```python
from build123d import *

# Parameters (mm, degrees)
F0_W     = 47.244
F0_H     = 31.496
F1_DEPTH = 3.20802
F2_R     = 2.4638
F3_DEPTH = 1.7526


with BuildPart() as f1:
    # F0 (on Top) → F1 (new body)
    with BuildSketch(Plane.XY):
        Rectangle(F0_W, F0_H)
    extrude(amount=F1_DEPTH)

    # F2 (on face) → F3 (join)
    with BuildSketch(Plane.XY.offset(3.20802)):
        with BuildLine():
            ThreePointArc((-17.2212, 11.811), (-21.4271696875, 13.5531696875), (-19.685, 9.3472))
            ThreePointArc((-19.685, 9.3472), (-17.9428303125, 10.0688303125), (-17.2212, 11.811))
        make_face()
        with Locations((-11.811, 11.811)):
            Circle(F2_R)
        with BuildLine():
            Line((-3.937, 11.811), (-3.937, 9.3472))
            ThreePointArc((-3.937, 9.3472), (-2.1948303125, 10.0688303125), (-1.4732, 11.811))
            ThreePointArc((-1.4732, 11.811), (-3.937, 14.2748), (-6.4008, 11.811))
            Line((-6.4008, 11.811), (-3.937, 11.811))
        make_face()
        with BuildLine():
            ThreePointArc((-6.4008, 11.811), (-5.6791696875, 10.0688303125), (-3.937, 9.3472))
            Line((-3.937, 9.3472), (-3.937, 11.811))
            Line((-3.937, 11.811), (-6.4008, 11.811))
        make_face()
        with BuildLine():
            ThreePointArc((6.4008, 11.811), (2.1948303125, 13.5531696875), (3.937, 9.3472))
            Line((3.937, 9.3472), (3.937, 11.811))
            Line((3.937, 11.811), (6.4008, 11.811))
        make_face()
        with BuildLine():
            Line((3.937, 11.811), (3.937, 9.3472))
            ThreePointArc((3.937, 9.3472), (5.6791696875, 10.0688303125), (6.4008, 11.811))
            Line((6.4008, 11.811), (3.937, 11.811))
        make_face()
        with BuildLine():
            Line((3.937, 3.937), (3.937, 1.4732))
            ThreePointArc((3.937, 1.4732), (5.6791696875, 2.1948303125), (6.4008, 3.937))
            ThreePointArc((6.4008, 3.937), (5.6791696875, 5.6791696875), (3.937, 6.4008))
            Line((3.937, 6.4008), (3.937, 3.937))
        make_face()
        with BuildLine():
            ThreePointArc((3.937, 6.4008), (1.4732, 3.937), (3.937, 1.4732))
            Line((3.937, 1.4732), (3.937, 3.937))
            Line((3.937, 3.937), (3.937, 6.4008))
        make_face()
        with BuildLine():
            Line((-3.937, 3.937), (-6.4008, 3.937))
            ThreePointArc((-6.4008, 3.937), (-3.937, 1.4732), (-1.4732, 3.937))
            ThreePointArc((-1.4732, 3.937), (-2.1948303125, 5.6791696875), (-3.937, 6.4008))
            Line((-3.937, 6.4008), (-3.937, 3.937))
        make_face()
        with BuildLine():
            ThreePointArc((-3.937, 6.4008), (-5.6791696875, 5.6791696875), (-6.4008, 3.937))
            Line((-6.4008, 3.937), (-3.937, 3.937))
            Line((-3.937, 3.937), (-3.937, 6.4008))
        make_face()
        with BuildLine():
            ThreePointArc((-9.3472, 3.937), (-11.811, 6.4008), (-14.2748, 3.937))
            Line((-14.2748, 3.937), (-11.811, 3.937))
            Line((-11.811, 3.937), (-9.3472, 3.937))
        make_face()
        with BuildLine():
            Line((-11.811, 3.937), (-14.2748, 3.937))
            ThreePointArc((-14.2748, 3.937), (-11.811, 1.4732), (-9.3472, 3.937))
            Line((-9.3472, 3.937), (-11.811, 3.937))
        make_face()
        with BuildLine():
            Line((-19.685, 6.4008), (-19.685, 3.937))
            Line((-19.685, 3.937), (-17.2212, 3.937))
            ThreePointArc((-17.2212, 3.937), (-17.9428303125, 5.6791696875), (-19.685, 6.4008))
        make_face()
        with BuildLine():
            Line((-19.685, 3.937), (-19.685, 1.4732))
            ThreePointArc((-19.685, 1.4732), (-17.9428303125, 2.1948303125), (-17.2212, 3.937))
            Line((-17.2212, 3.937), (-19.685, 3.937))
        make_face()
        with BuildLine():
            ThreePointArc((-19.685, 6.4008), (-22.1488, 3.937), (-19.685, 1.4732))
            Line((-19.685, 1.4732), (-19.685, 3.937))
            Line((-19.685, 3.937), (-19.685, 6.4008))
        make_face()
        with BuildLine():
            ThreePointArc((-17.2212, -3.937), (-17.9428303125, -2.1948303125), (-19.685, -1.4732))
            Line((-19.685, -1.4732), (-19.685, -3.937))
            Line((-19.685, -3.937), (-17.2212, -3.937))
        make_face()
        with BuildLine():
            Line((-17.2212, -3.937), (-19.685, -3.937))
            Line((-19.685, -3.937), (-19.685, -6.4008))
            ThreePointArc((-19.685, -6.4008), (-17.9428303125, -5.6791696875), (-17.2212, -3.937))
        make_face()
        with BuildLine():
            Line((-19.685, -3.937), (-19.685, -1.4732))
            ThreePointArc((-19.685, -1.4732), (-22.1488, -3.937), (-19.685, -6.4008))
            Line((-19.685, -6.4008), (-19.685, -3.937))
        make_face()
        with BuildLine():
            ThreePointArc((-9.3472, -3.937), (-11.811, -1.4732), (-14.2748, -3.937))
            Line((-14.2748, -3.937), (-11.811, -3.937))
            Line((-11.811, -3.937), (-9.3472, -3.937))
        make_face()
        with BuildLine():
            Line((-11.811, -3.937), (-14.2748, -3.937))
            ThreePointArc((-14.2748, -3.937), (-11.811, -6.4008), (-9.3472, -3.937))
            Line((-9.3472, -3.937), (-11.811, -3.937))
        make_face()
        with BuildLine():
            Line((-3.937, -3.937), (-6.4008, -3.937))
            ThreePointArc((-6.4008, -3.937), (-5.6791696875, -5.6791696875), (-3.937, -6.4008))
            Line((-3.937, -6.4008), (-3.937, -3.937))
        make_face()
        with BuildLine():
            ThreePointArc((-1.4732, -3.937), (-3.937, -1.4732), (-6.4008, -3.937))
            Line((-6.4008, -3.937), (-3.937, -3.937))
            Line((-3.937, -3.937), (-3.937, -6.4008))
            ThreePointArc((-3.937, -6.4008), (-2.1948303125, -5.6791696875), (-1.4732, -3.937))
        make_face()
        with BuildLine():
            ThreePointArc((-1.4732, -11.811), (-2.1948303125, -10.0688303125), (-3.937, -9.3472))
            Line((-3.937, -9.3472), (-3.937, -11.811))
            Line((-3.937, -11.811), (-6.4008, -11.811))
            ThreePointArc((-6.4008, -11.811), (-3.937, -14.2748), (-1.4732, -11.811))
        make_face()
        with BuildLine():
            Line((-3.937, -11.811), (-3.937, -9.3472))
            ThreePointArc((-3.937, -9.3472), (-5.6791696875, -10.0688303125), (-6.4008, -11.811))
            Line((-6.4008, -11.811), (-3.937, -11.811))
        make_face()
        with Locations((-11.811, -11.811)):
            Circle(F2_R)
        with BuildLine():
            ThreePointArc((-17.2212, -11.811), (-17.9428303125, -10.0688303125), (-19.685, -9.3472))
            ThreePointArc((-19.685, -9.3472), (-21.4271696875, -13.5531696875), (-17.2212, -11.811))
        make_face()
        with BuildLine():
            Line((3.937, -11.811), (3.937, -9.3472))
            ThreePointArc((3.937, -9.3472), (2.1948303125, -13.5531696875), (6.4008, -11.811))
            Line((6.4008, -11.811), (3.937, -11.811))
        make_face()
        with BuildLine():
            ThreePointArc((6.4008, -11.811), (5.6791696875, -10.0688303125), (3.937, -9.3472))
            Line((3.937, -9.3472), (3.937, -11.811))
            Line((3.937, -11.811), (6.4008, -11.811))
        make_face()
        with BuildLine():
            ThreePointArc((6.4008, -3.937), (5.6791696875, -2.1948303125), (3.937, -1.4732))
            Line((3.937, -1.4732), (3.937, -3.937))
            Line((3.937, -3.937), (3.937, -6.4008))
            ThreePointArc((3.937, -6.4008), (5.6791696875, -5.6791696875), (6.4008, -3.937))
        make_face()
        with BuildLine():
            Line((3.937, -3.937), (3.937, -1.4732))
            ThreePointArc((3.937, -1.4732), (1.4732, -3.937), (3.937, -6.4008))
            Line((3.937, -6.4008), (3.937, -3.937))
        make_face()
        with Locations((11.811, -3.937)):
            Circle(F2_R)
        with BuildLine():
            Line((19.685, -3.937), (19.685, -6.4008))
            ThreePointArc((19.685, -6.4008), (21.4271696875, -5.6791696875), (22.1488, -3.937))
            ThreePointArc((22.1488, -3.937), (19.685, -1.4732), (17.2212, -3.937))
            Line((17.2212, -3.937), (19.685, -3.937))
        make_face()
        with BuildLine():
            ThreePointArc((17.2212, -3.937), (17.9428303125, -5.6791696875), (19.685, -6.4008))
            Line((19.685, -6.4008), (19.685, -3.937))
            Line((19.685, -3.937), (17.2212, -3.937))
        make_face()
        with BuildLine():
            Line((19.685, -11.811), (17.2212, -11.811))
            ThreePointArc((17.2212, -11.811), (19.685, -14.2748), (22.1488, -11.811))
            ThreePointArc((22.1488, -11.811), (21.4271696875, -10.0688303125), (19.685, -9.3472))
            Line((19.685, -9.3472), (19.685, -11.811))
        make_face()
        with BuildLine():
            ThreePointArc((19.685, -9.3472), (17.9428303125, -10.0688303125), (17.2212, -11.811))
            Line((17.2212, -11.811), (19.685, -11.811))
            Line((19.685, -11.811), (19.685, -9.3472))
        make_face()
        with BuildLine():
            ThreePointArc((14.2748, -11.811), (11.811, -9.3472), (9.3472, -11.811))
            Line((9.3472, -11.811), (11.811, -11.811))
            Line((11.811, -11.811), (14.2748, -11.811))
        make_face()
        with BuildLine():
            Line((11.811, -11.811), (9.3472, -11.811))
            ThreePointArc((9.3472, -11.811), (11.811, -14.2748), (14.2748, -11.811))
            Line((14.2748, -11.811), (11.811, -11.811))
        make_face()
        with BuildLine():
            ThreePointArc((22.1488, 3.937), (21.4271696875, 5.6791696875), (19.685, 6.4008))
            Line((19.685, 6.4008), (19.685, 3.937))
            Line((19.685, 3.937), (17.2212, 3.937))
            ThreePointArc((17.2212, 3.937), (19.685, 1.4732), (22.1488, 3.937))
        make_face()
        with BuildLine():
            Line((19.685, 3.937), (19.685, 6.4008))
            ThreePointArc((19.685, 6.4008), (17.9428303125, 5.6791696875), (17.2212, 3.937))
            Line((17.2212, 3.937), (19.685, 3.937))
        make_face()
        with Locations((11.811, 3.937)):
            Circle(F2_R)
        with BuildLine():
            Line((11.811, 11.811), (9.3472, 11.811))
            ThreePointArc((9.3472, 11.811), (11.811, 9.3472), (14.2748, 11.811))
            Line((14.2748, 11.811), (11.811, 11.811))
        make_face()
        with BuildLine():
            ThreePointArc((14.2748, 11.811), (11.811, 14.2748), (9.3472, 11.811))
            Line((9.3472, 11.811), (11.811, 11.811))
            Line((11.811, 11.811), (14.2748, 11.811))
        make_face()
        with BuildLine():
            ThreePointArc((22.1488, 11.811), (19.685, 14.2748), (17.2212, 11.811))
            Line((17.2212, 11.811), (19.685, 11.811))
            Line((19.685, 11.811), (19.685, 9.3472))
            ThreePointArc((19.685, 9.3472), (21.4271696875, 10.0688303125), (22.1488, 11.811))
        make_face()
        with BuildLine():
            Line((19.685, 11.811), (17.2212, 11.811))
            ThreePointArc((17.2212, 11.811), (17.9428303125, 10.0688303125), (19.685, 9.3472))
            Line((19.685, 9.3472), (19.685, 11.811))
        make_face()
    extrude(amount=F3_DEPTH)


solid = f1.part
```
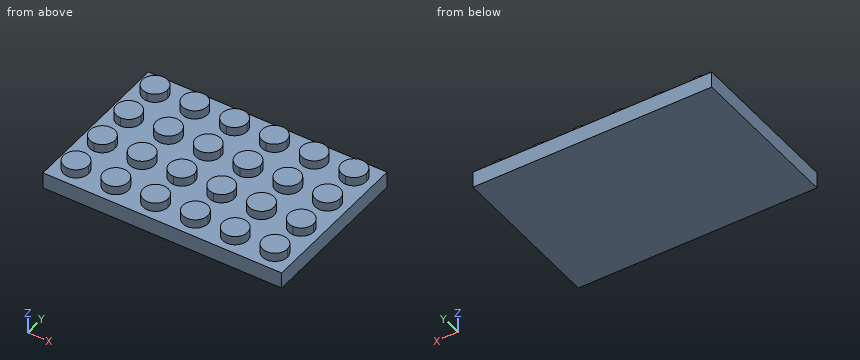
Here's how the part is built. I have some questions about the finished solid (model axes, mm). Give positions to 0.01 mm unless a question says otherwise; leave off trailing zeros. Order: outer loops, then holes, each group sorted by start corner. A loop starts at its lowest first (then second) coordinate and runs counter-clockwise, first axis right, second up. Notation, with made-up numbers: M -24.5,15.25 L -4.5,15.25 A22 ccw -4.5,50.25 Z; hole C 5,19.5 d7. An arc over 180 degrees is marked long. Use a Markdown table: item, result. Add a question column.
1. I need wall thicknesses on probe 1 along X at (y, z) = (12, 4.25); probe 2 along X at (y, z) = (-10, 4.5); probe 3 along Y at (x, z) = (-19, 3.3). Which ranges of each line are inside material? Lowest first, please. Write a range as from..to.
2. Suppose I cut it at D-D (x = -10). List the corners of the cut face in (y, z) for me, and give its area (3 significant figures).
3. Suppose I cut it at B-B (z = 3.9). Give the number of separate pieces and of enclosed holes in the cut face, and give its area (3 significant figures).
4. Suppose I cut it at C-C (y = -5). List the corners of the cut face in (x, z) for me, and give its area (3 significant figures).
5. Suppose I cut it at A-A (x = -3). List the corners of the cut face in (y, z) for me, and give its area (3 significant figures).
Results list:
| question | item | result |
|---|---|---|
| 1 | probe 1 | x = -22.14..-17.23, -14.27..-9.35, -6.39..-1.48, 1.48..6.39, 9.35..14.27, 17.23..22.14 |
| 1 | probe 2 | x = -21.36..-18.01, -13.48..-10.14, -5.61..-2.27, 2.27..5.61, 10.14..13.48, 18.01..21.36 |
| 1 | probe 3 | y = -14.18..-9.44, -6.3..-1.57, 1.57..6.3, 9.44..14.18 |
| 2 | outline | M -15.75,0 L 15.75,0 L 15.75,3.21 L 13.48,3.21 L 13.48,4.96 L 10.14,4.96 L 10.14,3.21 L 5.61,3.21 L 5.61,4.96 L 2.27,4.96 L 2.27,3.21 L -2.27,3.21 L -2.27,4.96 L -5.61,4.96 L -5.61,3.21 L -10.14,3.21 L -10.14,4.96 L -13.48,4.96 L -13.48,3.21 L -15.75,3.21 Z |
| 2 | area | 124 mm² |
| 3 | separate pieces | 24 |
| 3 | enclosed holes | 0 |
| 3 | area | 458 mm² |
| 4 | outline | M -23.62,0 L 23.62,0 L 23.62,3.21 L 21.91,3.21 L 21.91,4.96 L 17.46,4.96 L 17.46,3.21 L 14.03,3.21 L 14.03,4.96 L 9.59,4.96 L 9.59,3.21 L 6.16,3.21 L 6.16,4.96 L 1.71,4.96 L 1.71,3.21 L -1.71,3.21 L -1.71,4.96 L -6.16,4.96 L -6.16,3.21 L -9.59,3.21 L -9.59,4.96 L -14.03,4.96 L -14.03,3.21 L -17.46,3.21 L -17.46,4.96 L -21.91,4.96 L -21.91,3.21 L -23.62,3.21 Z |
| 4 | area | 198 mm² |
| 5 | outline | M -15.75,0 L 15.75,0 L 15.75,3.21 L 14.09,3.21 L 14.09,4.96 L 9.53,4.96 L 9.53,3.21 L 6.22,3.21 L 6.22,4.96 L 1.66,4.96 L 1.66,3.21 L -1.66,3.21 L -1.66,4.96 L -6.22,4.96 L -6.22,3.21 L -9.53,3.21 L -9.53,4.96 L -14.09,4.96 L -14.09,3.21 L -15.75,3.21 Z |
| 5 | area | 133 mm² |
